from build123d import *

# Parameters (mm, degrees)
SKETCH_1_W          = 70
SKETCH_1_H          = 30
EXTRUDE_1_DEPTH     = 30
SKETCH_2_R          = 1.6
CUT_EXTRUDE_1_DEPTH = 31
SKETCH_3_W          = 28.2
SKETCH_3_H          = 13.8
CUT_EXTRUDE_2_DEPTH = 31
EXTRUDE_2_DEPTH     = 1.2
SKETCH_5_R          = 1.1
CUT_EXTRUDE_3_DEPTH = 3.1
SKETCH_6_W          = 10
SKETCH_6_H          = 30
CUT_EXTRUDE_4_DEPTH = 20
SKETCH_7_R          = 1.8
CUT_EXTRUDE_5_DEPTH = 10.2
SKETCH_8_R          = 2.15
CUT_EXTRUDE_6_DEPTH = 0.8
SKETCH_9_R          = 1.8
CUT_EXTRUDE_7_DEPTH = 10.2
SKETCH_10_R         = 2.15
CUT_EXTRUDE_8_DEPTH = 0.8
FILLET_1_R          = 2
FILLET_2_R          = 1


with BuildPart() as part:
    # 草图1 → 凸台-拉伸1 (new body)
    with BuildSketch(Plane.XY):
        with Locations((35, 15)):
            Rectangle(SKETCH_1_W, SKETCH_1_H)
    extrude(amount=EXTRUDE_1_DEPTH)

    # 草图2 → 切除-拉伸1 (cut, through all)
    with BuildSketch(Plane.XY.offset(30)):
        with Locations((5, 5)):
            Circle(SKETCH_2_R)
        with Locations((65, 5)):
            Circle(SKETCH_2_R)
        with Locations((65, 25)):
            Circle(SKETCH_2_R)
        with Locations((5, 25)):
            Circle(SKETCH_2_R)
    extrude(amount=-CUT_EXTRUDE_1_DEPTH, mode=Mode.SUBTRACT)

    # 草图3 → 切除-拉伸2 (cut, through all)
    with BuildSketch(Plane.XZ):
        with Locations((35, 10)):
            Rectangle(SKETCH_3_W, SKETCH_3_H)
    extrude(amount=-CUT_EXTRUDE_2_DEPTH, mode=Mode.SUBTRACT)

    # 草图4 → 凸台-拉伸2 (add)
    with BuildSketch(Plane.XZ):
        with BuildLine():
            ThreePointArc((20.9, 10), (22.92096321, 14.87903679), (27.8, 16.9))
            Line((27.8, 16.9), (20.9, 16.9))
            Line((20.9, 16.9), (20.9, 10))
        make_face()
        with BuildLine():
            ThreePointArc((27.8, 3.1), (22.92096321, 5.12096321), (20.9, 10))
            Line((20.9, 10), (20.9, 3.1))
            Line((20.9, 3.1), (27.8, 3.1))
        make_face()
        with BuildLine():
            Line((49.1, 16.9), (42.2, 16.9))
            ThreePointArc((42.2, 16.9), (47.079036757, 14.879036823), (49.1, 10.000000094))
            Line((49.1, 10.000000094), (49.1, 16.9))
        make_face()
        with BuildLine():
            Line((49.1, 3.1), (49.1, 10.000000094))
            ThreePointArc((49.1, 10.000000094), (47.079036823, 5.120963243), (42.2, 3.1))
            Line((42.2, 3.1), (49.1, 3.1))
        make_face()
    extrude(amount=-EXTRUDE_2_DEPTH)

    # 草图5 → 切除-拉伸3 (cut)
    with BuildSketch(Plane(origin=(0, 0, 0), x_dir=(-1, 0, 0), z_dir=(0, 0, -1))):
        with Locations((-45.8, 11.1)):
            Circle(SKETCH_5_R)
        with Locations((-24.2, 11.1)):
            Circle(SKETCH_5_R)
    extrude(amount=-CUT_EXTRUDE_3_DEPTH, mode=Mode.SUBTRACT)

    # 草图6 → 切除-拉伸4 (cut)
    with BuildSketch(Plane(origin=(0, 0, 0), x_dir=(-1, 0, 0), z_dir=(0, 0, -1))):
        with Locations((-65, 15)):
            Rectangle(SKETCH_6_W, SKETCH_6_H)
        with Locations((-5, 15)):
            Rectangle(SKETCH_6_W, SKETCH_6_H)
    extrude(amount=-CUT_EXTRUDE_4_DEPTH, mode=Mode.SUBTRACT)

    # 草图7 → 切除-拉伸5 (cut)
    with BuildSketch(Plane.XZ):
        with Locations((54, 10)):
            Circle(SKETCH_7_R)
        with Locations((16, 10)):
            Circle(SKETCH_7_R)
        with Locations((54, 25)):
            Circle(SKETCH_7_R)
        with Locations((16, 25)):
            Circle(SKETCH_7_R)
    extrude(amount=-CUT_EXTRUDE_5_DEPTH, mode=Mode.SUBTRACT)

    # 草图8 → 切除-拉伸6 (cut)
    with BuildSketch(Plane.XZ):
        with Locations((54, 10)):
            Circle(SKETCH_8_R)
        with Locations((16, 10)):
            Circle(SKETCH_8_R)
        with Locations((54, 25)):
            Circle(SKETCH_8_R)
        with Locations((16, 25)):
            Circle(SKETCH_8_R)
    extrude(amount=-CUT_EXTRUDE_6_DEPTH, mode=Mode.SUBTRACT)

    # 草图9 → 切除-拉伸7 (cut)
    with BuildSketch(Plane(origin=(0, 0, 0), x_dir=(-1, 0, 0), z_dir=(0, 0, -1))):
        with Locations((-54, 23)):
            Circle(SKETCH_9_R)
        with Locations((-16, 23)):
            Circle(SKETCH_9_R)
    extrude(amount=-CUT_EXTRUDE_7_DEPTH, mode=Mode.SUBTRACT)

    # 草图10 → 切除-拉伸8 (cut)
    with BuildSketch(Plane(origin=(0, 0, 0), x_dir=(-1, 0, 0), z_dir=(0, 0, -1))):
        with Locations((-54, 23)):
            Circle(SKETCH_10_R)
        with Locations((-16, 23)):
            Circle(SKETCH_10_R)
    extrude(amount=-CUT_EXTRUDE_8_DEPTH, mode=Mode.SUBTRACT)

    # 圆角1
    fillet_1_edges = [part.edges().sort_by_distance(p)[0] for p in [
        (60, 15, 0),
        (70, 15, 20),
        (60, 15, 20),
        (10, 15, 0),
        (10, 15, 20),
        (0, 15, 20),
    ]]
    fillet(fillet_1_edges, radius=FILLET_1_R)

    # 圆角2
    fillet_2_edges = [part.edges().sort_by_distance(p)[0] for p in [
        (20.9, 15.6, 3.1),
        (20.9, 15.6, 16.9),
        (49.1, 15.6, 16.9),
        (49.1, 15.6, 3.1),
    ]]
    fillet(fillet_2_edges, radius=FILLET_2_R)


solid = part.part
Design review of the part built by this model. Coordinates are the model's own, in mm. A direction names the side the tool comes from. Coordinates: 2 decimals unless noted, no trailing zeros. Write each loop counter-clockwise with the first axis right and the second up, starting at its lowest first coordinate (ties: lowest second). Pieces come first, ordered by that corner, then holes. Notation, with made-up numbers: (29, -32.75) - (55, -32.75) arc R15 ccw to (55, -13.75) - close; hole circle Ø9 at (-32, -8). An arc over 180 degrees is marked (long way). Use one line per item in the form item = value.
Q1. For probe 1 along Z at (x, y) = (16, 0.4); probe 2 along Y at (x, z) = (65, 25.25); probe 3 along Z at (x, y) = (42, 12.5), list the stretches that pass through material, from the lowest coordinate up.
Taken from the geometry:
probe_1 = 0 to 7.85, 12.15 to 22.85, 27.15 to 30
probe_2 = 0 to 3.4, 6.6 to 23.4, 26.6 to 30
probe_3 = 0 to 3.1, 16.9 to 30
Q2. Consider section D-D (y = 14.5). Write out the cut boundary in (x, z), plus the area to 3 significant figures.
Taken from the geometry:
outline = (0, 22) arc R2 ccw to (2, 20) - (8, 20) arc R2 cw to (10, 18) - (10, 2) arc R2 ccw to (12, 0) - (58, 0) arc R2 ccw to (60, 2) - (60, 18) arc R2 cw to (62, 20) - (68, 20) arc R2 ccw to (70, 22) - (70, 30) - (0, 30) - close; hole (20.9, 4.1) arc R1 ccw to (21.9, 3.1) - (48.1, 3.1) arc R1 ccw to (49.1, 4.1) - (49.1, 15.9) arc R1 ccw to (48.1, 16.9) - (21.9, 16.9) arc R1 ccw to (20.9, 15.9) - close
area = 1,310 mm^2
Q3. Consider section B-B (x = 5). Write out the cut boundary in (y, z).
Taken from the geometry:
outline = (0, 20) - (3.4, 20) - (3.4, 30) - (0, 30) - close; (6.6, 20) - (23.4, 20) - (23.4, 30) - (6.6, 30) - close; (26.6, 20) - (30, 20) - (30, 30) - (26.6, 30) - close
Q4. Machinability: for faces 4 (the flat face through (5, 15, 20)), 5 (the flat face through (35, 15, 3.1)), 6 (the flat face through (60, 15, 10)), 7 (the flat face through (54, 0.8, 8)), which of the approach directions +Z, -Z, +X, -X, +Y, -Y give a long, thin tool a straight path to every point of the face, cutting with its end or side? Answer none if there is none.
Taken from the geometry:
face_4 = -Z, -X, +Y, -Y
face_5 = +Y
face_6 = -Z, +X, +Y, -Y
face_7 = -Y
Q5. Consider section A-A (y = 5). Count the separate pieces of the cut face and the enclosed holes in it, plus the area to 3 significant figures.
Taken from the geometry:
separate_pieces = 3
enclosed_holes = 5
area = 1,210 mm^2
Q6. The part is to be moulded in two halves that separate along X. For faces 1 (the flat face through (22, 1.2, 5)), 2 (the flat face through (10, 15, 10)), 3 (the cylindrical face through (59.4, 15.21, 0.57)), say which applies: +X half, -X half, draft (parallel to the pull), parting line (faces both ways), or undercut.
Taken from the geometry:
face_1 = undercut
face_2 = -X half
face_3 = +X half
Q7. Insertion check: pin 1 Ø1.8 at (x, z) = (15.5, 24.5) entering from -Y; pin 2 Ø3.5 at (x, y) = (5, 5) entering from -Z; pin 3 Ø1.1 at (x, y) = (15.5, 23) entering from -Z. Each pin has a flat end and moves straight along its axis. Give the tip position at first contact, or say it passes through.
Taken from the geometry:
pin_1 = 10.2
pin_2 = 20
pin_3 = 10.2
